Here's how the part is built. I have some questions about the finished solid (model axes, mm). A direction names the side the tool comes from. Round coordinates to 2 decimals unless told otherwise and drop trailing zeros. Order: outer loops, then holes, each group sorted by start corner. A loop starts at its lowest first (then second) coordinate and runs counter-clockwise, first axis right, second up. Notation, with made-up numbers: (26.25, 76) - (38.25, 76) arc R21 ccw to (38.25, 109) - close; hole circle Ø10 at (-11, 83.25). An arc over 180 degrees is marked (long way). Answer as a JSON object with one key per item and string values.
```python
from build123d import *

# Parameters (mm, degrees)
EXTRUDE_419_DEPTH      = 8.8
FILLET_1296_R          = 0.6
PATTERN_LINEAR_1_COUNT = 18
PATTERN_LINEAR_1_PITCH = 2
HOLE_WIZARD_6_0_6_1_D  = 6
M8X1_0_1_D             = 7
M8X1_0_1_DEPTH         = 13
M8X1_0_1_TIP           = 2.103012167


with BuildPart() as part:
    # 草图1 → Extrude 419 (new body)
    with BuildSketch(Plane(origin=(0, 0, 0), x_dir=(0, 0, -1), z_dir=(1, 0, 0))):
        Polygon((10.5, 6.062177826), (10.5, -6.062177826), (0, -12.124355653), (-10.5, -6.062177826), (-10.5, 6.062177826), (0, 12.124355653), align=None)
    extrude(amount=EXTRUDE_419_DEPTH)

    # 草图2 → 凸台-旋转1 (revolve)
    with BuildSketch(Plane.XY, mode=Mode.PRIVATE) as revolve_1_sk:
        Polygon((0, 0), (58.8, 0), (58.8, 5.268), (58.8, 7), (0, 7), align=None)
    revolve(revolve_1_sk.sketch.rotate(Axis((0, 0, 0), (1, 0, 0)), 90), axis=Axis((0, 0, 0), (1, 0, 0)))

    # 草图3 → 切除-旋转1 (revolve, cut)
    with BuildSketch(Plane.XY):
        Polygon((0, 10.5), (3.824573519, 17.124355653), (3.824573519, 22.124355653), (-10, 22.124355653), (-10, 10.5), align=None)
    revolve(axis=Axis((0, 0, 0), (1, 0, 0)), mode=Mode.SUBTRACT)

    # 草图4 → 切除-旋转3 (revolve, cut)
    with BuildSketch(Plane.XY, mode=Mode.PRIVATE) as cut_revolve_3_sk:
        Polygon((8.8, 9.82), (8.2, 10.166410162), (8.2, 12.124355653), (8.8, 12.124355653), align=None)
    revolve(cut_revolve_3_sk.sketch.rotate(Axis((0, 0, 0), (1, 0, 0)), 90), axis=Axis((0, 0, 0), (1, 0, 0)), mode=Mode.SUBTRACT)

    # Fillet 1296
    fillet_1296_edges = [part.edges().sort_by_distance(p)[0] for p in [
        (8.8, 0, -7),
    ]]
    fillet(fillet_1296_edges, radius=FILLET_1296_R)

    # 草图6 → 切除-旋转4 (revolve, cut)
    with BuildSketch(Plane.XY, mode=Mode.PRIVATE) as cut_revolve_4_sk:
        Polygon((57.8, 7), (59.8, 7), (58.8, 5.267949192), align=None)
    cut_revolve_4 = revolve(cut_revolve_4_sk.sketch.rotate(Axis((0, 0, 0), (1, 0, 0)), 90), axis=Axis((0, 0, 0), (1, 0, 0)), mode=Mode.SUBTRACT)

    # 阵列(线性)1: 切除-旋转4 ×18
    with Locations(*[(-i * PATTERN_LINEAR_1_PITCH, 0, 0) for i in range(1, PATTERN_LINEAR_1_COUNT)]):
        add(cut_revolve_4, mode=Mode.SUBTRACT)

    # Ø6.0 (6) 直径孔1 (through all)
    with Locations(Plane(origin=(0, 0, 0), x_dir=(0, 0, -1), z_dir=(-1, 0, 0))):
        with Locations((0, 0)):
            Hole(HOLE_WIZARD_6_0_6_1_D / 2)

    # M8x1.0 螺纹孔1
    with Locations(Plane(origin=(0, 0, 0), x_dir=(0, 0, -1), z_dir=(-1, 0, 0))):
        with Locations((0, 0)):
            Hole(M8X1_0_1_D / 2, depth=M8X1_0_1_DEPTH)
            with Locations((0, 0, -(M8X1_0_1_DEPTH + M8X1_0_1_TIP / 2))):  # 118° drill point
                Cone(0, M8X1_0_1_D / 2, M8X1_0_1_TIP, mode=Mode.SUBTRACT)


solid = part.part
```
1. If I drill on L1, parallel to Y at x = 10, z = 0; L2, parallel to Y at x = 5, z = 0; L3, parallel to X at y = 6.25, z = -8.25, over which ranges is the centre line in solid material (lowest first)? Write a range as [from, to].
Responses:
{"L1": "[-7, -3.5], [3.5, 7]", "L2": "[-12.12, -3.5], [3.5, 12.12]", "L3": "[0, 8.2]"}
2. Thinking about a two-plate mould opening in Y: for faces 1 (the face through (36, 0, -3)), 2 (the face through (0.228, 10.895, -0.027)), 3 (the face through (16.5, 6.21, 3.23)), which applies, pulls with the +Y half, pulls with the -Y half, needs draft (parallel to the pull), parting line crosses it, or undercut?
Responses:
{"face 1": "undercut", "face 2": "pulls with the +Y half", "face 3": "parting line crosses it"}
3. For faces 4 (the face through (6.591, 1.341, 3.233)), 5 (the face through (8.2, 10, 3)), which set-ups out of +Z, -Z, +X, -X, +Y, -Y let a thin tool reach every point of the face, with its end or its side?
Responses:
{"face 4": "-X", "face 5": "+X"}
4. For P1, Ø6, axis at x = 14.5, y = 4, coming from the -Z side; P2, Ø8, axis at x = 27, y = 9.5, coming from the +Z side; P3, Ø1.5, axis at x = 42, y = -0.5, coming from the -Z side; P4, Ø4, axis at y = 0, z = 0, coming from the +X side, each with a flat end and sliding along its axis, tell me the tip position at first contact or that it passes through.
Responses:
{"P1": "z = -6.93", "P2": "z = 4.23", "P3": "z = -7", "P4": "through"}
5. Imagine slicing it at A-A (x = 14). List the corners of the cut face in (y, z) for me, plus the area to 3 significant figures.
Responses:
{"outline": "circle Ø14 at (0, 0); hole circle Ø6 at (0, 0)", "area": "126 mm2"}
